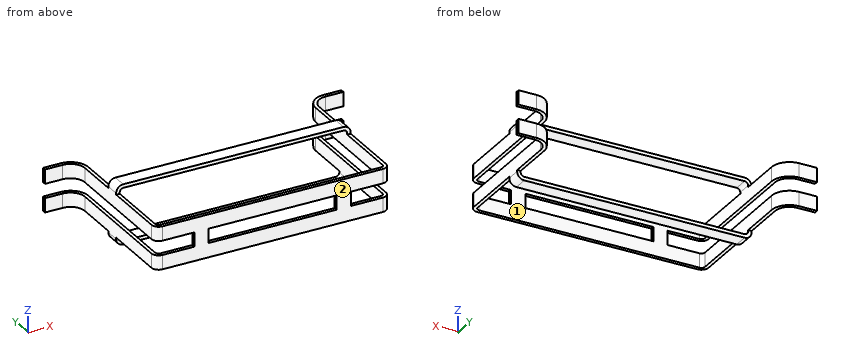
from build123d import *

# Parameters (mm, degrees)
EXTRUDE_1_DEPTH   = 20
EXTRUDE_2_DEPTH   = 20
SKETCH_3_W        = 20
SKETCH_3_H        = 20
EXTRUDE_1_2_DEPTH = 5


with BuildPart() as part:
    # 草图1 → Extrude 1 (new body)
    with BuildSketch(Plane.XY):
        with BuildLine():
            Line((210, 200), (185, 200))
            ThreePointArc((185, 200), (170.857864376, 194.142135624), (165, 180))
            Line((165, 180), (165, 10))
            ThreePointArc((165, 10), (162.071067812, 2.928932188), (155, 0))
            Line((155, 0), (-155, 0))
            ThreePointArc((-155, 0), (-162.071067812, 2.928932188), (-165, 10))
            Line((-165, 10), (-165, 180))
            ThreePointArc((-165, 180), (-170.857864376, 194.142135624), (-185, 200))
            Line((-185, 200), (-210, 200))
            Line((-210, 200), (-210, 205))
            Line((-210, 205), (-185, 205))
            ThreePointArc((-185, 205), (-167.32233047, 197.67766953), (-160, 180))
            Line((-160, 180), (-160, 10))
            ThreePointArc((-160, 10), (-158.535533906, 6.464466094), (-155, 5))
            Line((-155, 5), (155, 5))
            ThreePointArc((155, 5), (158.535533906, 6.464466094), (160, 10))
            Line((160, 10), (160, 180))
            ThreePointArc((160, 180), (167.32233047, 197.67766953), (185, 205))
            Line((185, 205), (210, 205))
            Line((210, 205), (210, 200))
        make_face()
    extrude(amount=EXTRUDE_1_DEPTH)

    # 草图2 → 拉伸-薄壁2 (add)
    with BuildSketch(Plane(origin=(0, 100, 0), x_dir=(1, 0, 0), z_dir=(0, 1, 0))):
        with BuildLine():
            Line((-165, -20), (-165, -22))
            ThreePointArc((-165, -22), (-162.071067812, -29.071067812), (-155, -32))
            Line((-155, -32), (155, -32))
            ThreePointArc((155, -32), (162.071067812, -29.071067812), (165, -22))
            Line((165, -22), (165, -20))
            Line((165, -20), (160, -20))
            Line((160, -20), (160, -22))
            ThreePointArc((160, -22), (158.535533906, -25.535533906), (155, -27))
            Line((155, -27), (-155, -27))
            ThreePointArc((-155, -27), (-158.535533906, -25.535533906), (-160, -22))
            Line((-160, -22), (-160, -20))
            Line((-160, -20), (-165, -20))
        make_face()
    extrude(amount=EXTRUDE_2_DEPTH)


with BuildPart() as body_2:
    # 镜向3: mirrored copy
    add(part.part.mirror(Plane.XY.offset(-10)))


with BuildPart() as part_1:
    add(part.part)

    add(body_2.part)  # Extrude 1 2 merges body 2
    # 草图3 → Extrude 1 2 (add)
    with BuildSketch(Plane(origin=(0, 5, 0), x_dir=(1, 0, 0), z_dir=(0, 1, 0))):
        with Locations((-100, 10)):
            Rectangle(SKETCH_3_W, SKETCH_3_H)
    extrude_1_2 = extrude(amount=-EXTRUDE_1_2_DEPTH)

    # 镜向4: Extrude 1 2 across plane
    add(extrude_1_2.mirror(Plane(origin=(0, 0, 0), x_dir=(0, 0, 1), z_dir=(1, 0, 0))))


solid = part_1.part
The listing builds one solid part. Answer for the finished solid, in the listing's coordinates (mm). Face numbers are marked on the shaded views. Coordinates: 2 decimals unless noted, no trailing zeros. Loops run counter-clockwise (first coordinate to the right, second up) from the corner with the lowest first, then second, coordinate; pieces in that order, holes last. Notation, with made-up numbers: (45, 29.5) -> (53, 29.5) arc R21 ccw to (53, 38.5) -> close; hole circle Ø8 at (-4.5, -35.5). An arc over 180 degrees is marked (long way). Write item = value, one per line. Start each with the question number.
1) A cutting plane is placed at B-B (y = 24). Give the vertices of the cut face in (x, z), then the cut area to 3 significant figures.
2) A cutting plane is placed at C-C (z = -28). Give the vertices of the cut face in (x, y).
3) Straight lines are drawn through the part: line 1 (Z direction, x = -164, y = 144); line 2 (X direction, y = 30, z = 10); line 3 (Z direction, x = -13.5, y = 115). For each, find the intervals that lie inside material, in ascending order. Write a range as from..to.
4) A cutting plane is placed at A-A (x = 102). Give the vertices of the cut face in (y, z), then the cut area to 3 significant figures.
5) The mould has two halves that part along X. Classify the marked faces 1 and 2: released by +X, released by -X, zero draft, split by the parting line, or undercut.
6) Given pin 1 Ø3 at (y, z) = (167.5, -37.5) entering from +X; pin 2 Ø1.5 at (x, y) = (16.5, 2.5) entering from +Z; pin 3 Ø18 at (x, z) = (8, -23.5) entering from +Y, each flat-ended and moving along its own axis, determine where each tip first touches the part or whether it passes through.
7) A cutting plane is placed at D-D (x = -146). Give the vertices of the cut face in (y, z).
Responses:
q1.outline = (-165, -40) -> (-160, -40) -> (-160, -20) -> (-165, -20) -> close; (-165, 0) -> (-160, 0) -> (-160, 20) -> (-165, 20) -> close; (160, -40) -> (165, -40) -> (165, -20) -> (160, -20) -> close; (160, 0) -> (165, 0) -> (165, 20) -> (160, 20) -> close
q1.area = 400 mm²
q2.outline = (-210, 200) -> (-185, 200) arc R20 cw to (-165, 180) -> (-165, 10) arc R10 ccw to (-155, 0) -> (155, 0) arc R10 ccw to (165, 10) -> (165, 180) arc R20 cw to (185, 200) -> (210, 200) -> (210, 205) -> (185, 205) arc R25 ccw to (160, 180) -> (160, 10) arc R5 cw to (155, 5) -> (-155, 5) arc R5 cw to (-160, 10) -> (-160, 180) arc R25 ccw to (-185, 205) -> (-210, 205) -> close
q3.line_1 = -40..-20, 0..20
q3.line_2 = -165..-160, 160..165
q3.line_3 = -52..-47, 27..32
q4.outline = (0, -40) -> (5, -40) -> (5, 20) -> (0, 20) -> close; (100, -52) -> (120, -52) -> (120, -47) -> (100, -47) -> close; (100, 27) -> (120, 27) -> (120, 32) -> (100, 32) -> close
q4.area = 500 mm²
q5.face_1 = undercut
q5.face_2 = zero draft
q6.pin_1 = 165
q6.pin_2 = 20
q6.pin_3 = 5
q7.outline = (0, -40) -> (5, -40) -> (5, -20) -> (0, -20) -> close; (0, 0) -> (5, 0) -> (5, 20) -> (0, 20) -> close; (100, -52) -> (120, -52) -> (120, -47) -> (100, -47) -> close; (100, 27) -> (120, 27) -> (120, 32) -> (100, 32) -> close
